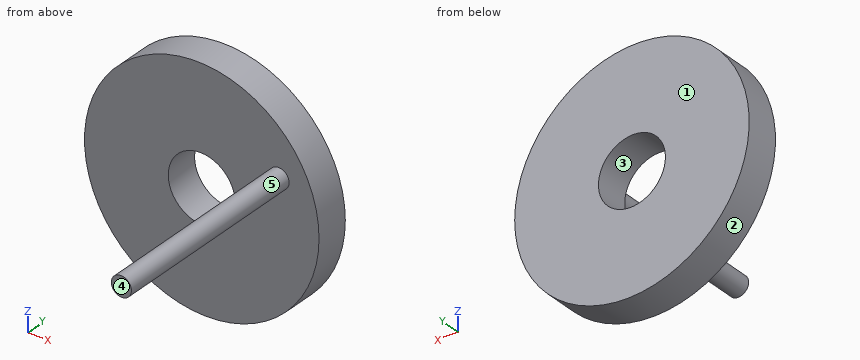
from build123d import *

# Parameters (mm, degrees)
F0_R     = 17.5
F1_DEPTH = 5
F2_R     = 1.5
F3_DEPTH = 30
F5_D     = 10


with BuildPart() as f1:
    # F0 (on Front) → F1 (new body)
    with BuildSketch(Plane.XZ):
        Circle(F0_R)
    extrude(amount=F1_DEPTH)

    # F2 (on face) → F3 (join)
    with BuildSketch(Plane.XZ.offset(5)):
        with Locations((11.532563, 6)):
            Circle(F2_R)
    extrude(amount=F3_DEPTH)

    # F5 (through all)
    with Locations(Plane(origin=(0, 0, 0), x_dir=(1, 0, 0), z_dir=(0, 1, 0))):
        with Locations((0, 0)):
            Hole(F5_D / 2)


solid = f1.part
Geometry check sheet. Reference: the model listing, model coordinates, mm. Face numbers are marked on the shaded views. A direction names the side the tool comes from. Round coordinates to 2 decimals unless told otherwise and drop trailing zeros. Write each loop counter-clockwise with the first axis right and the second up, starting at its lowest first coordinate (ties: lowest second). Pieces come first, ordered by that corner, then holes. Notation, with made-up numbers: (-34.5, -15) -> (-6.5, -15) arc R15 cw to (-6.5, -11) -> close; hole circle Ø11 at (-33.5, 83.5). An arc over 180 degrees is marked (long way). One line per item, written item: value. Start each with the question number.
(1) Cross-section at B-B, the plane x = 0. Record the cut outline in (y, z), and give its area (3 significant figures).
(2) Access from +Z, -Z, +X, -X, +Y, -Y to the whole of each face (thin tool, end or side, straight path). Record for the marked faces 4 and 5.
(3) Go/stop test with flat-tipped pins: pin 1 Ø10 at (x, z) = (-2, 9) entering from +Y; pin 2 Ø1 at (x, z) = (12.5, -13) entering from +Y; pin 3 Ø1 at (x, z) = (6, -3.5) entering from -Y; pin 4 Ø10 at (y, z) = (-31, 12) entering from -X. Record where each tip stops, or that it passes through.
(4) Cross-section at C-C, the plane y = -22. Record the cut outline in (x, z).
(5) Draft check along Z on the marked faces 1, 2 and 3. Enter one of: +Z half, -Z half, draft (parallel to the pull), parting line (faces both ways), or undercut.
(6) Cross-section at D-D, the plane z = 6. Record the cut outline in (x, y), and give its area (3 significant figures).
(7) Cross-section at A-A, the plane z = 0. Record the cut outline in (x, y), and give its area (3 significant figures).
(8) Scan lines: line 1 (Z direction, x = 0, y = -1.35); line 2 (Y direction, x = 7, z = 15); line 3 (X direction, y = -3, z = 1.5). Record each from-to range of solid material in increasing order. Write a range as [from, to].
Answer:
1. outline: (-5, -17.5) -> (0, -17.5) -> (0, -5) -> (-5, -5) -> close; (-5, 5) -> (0, 5) -> (0, 17.5) -> (-5, 17.5) -> close
1. area: 125 mm²
2. face 4: +Z, -Z, +X, -X, -Y
2. face 5: -Y
3. pin 1: y = 0
3. pin 2: through
3. pin 3: y = -5
3. pin 4: x = 10.41
4. outline: circle Ø3 at (11.53, 6)
5. face 1: draft
5. face 2: parting line
5. face 3: undercut
6. outline: (-16.44, -5) -> (10.03, -5) -> (10.03, -35) -> (13.03, -35) -> (13.03, -5) -> (16.44, -5) -> (16.44, 0) -> (-16.44, 0) -> close
6. area: 254 mm²
7. outline: (-17.5, -5) -> (-5, -5) -> (-5, 0) -> (-17.5, 0) -> close; (5, -5) -> (17.5, -5) -> (17.5, 0) -> (5, 0) -> close
7. area: 125 mm²
8. line 1: [-17.5, -5], [5, 17.5]
8. line 2: [-5, 0]
8. line 3: [-17.44, -4.77], [4.77, 17.44]
